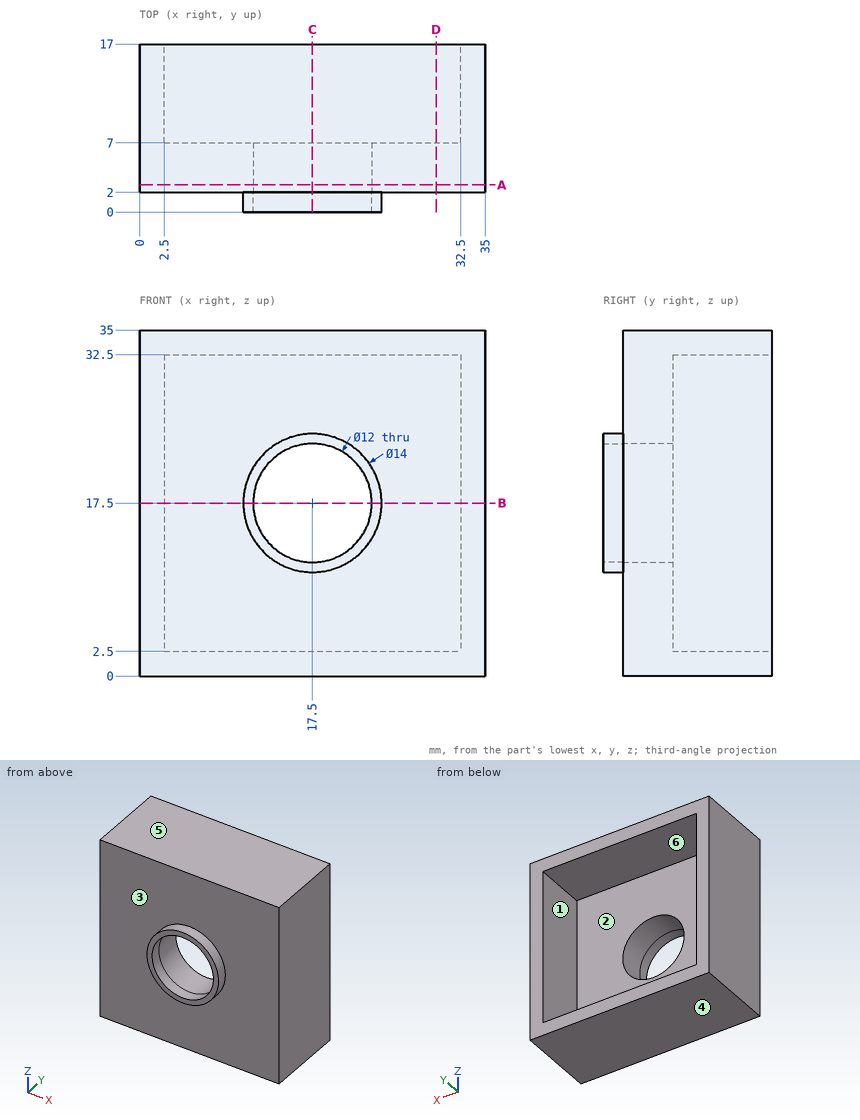
Print and shaded views of the part. All mm, measured from the part's lowest x, y and z. A direction names the side the tool comes from. Coordinates: 2 decimals unless noted, no trailing zeros. Order: outer loops, then holes, each group sorted by start corner. A loop starts at its lowest first (then second) coordinate and runs counter-clockwise, first axis right, second up. Notation, with made-up numbers: (-9.75, 31) -> (46.25, 31) arc R30 cw to (46.25, 54) -> close; hole circle Ø10 at (10, 88.25). An arc over 180 degrees is marked (long way). Answer as a JSON object with one key per item and string values. Group by question number.
1) Drill centre lines: L1, parallel to X at y = 12.25, z = 5.5; L2, parallel to X at y = 5.4, z = 17.5. Where is each one in solid material? Low to high.
2) Cut at D-D, the plane x = 30. Write the cut outline in (y, z), then the cut area to 3 significant figures.
3) Pull direction Z, two halves, no side cores. Call the marked faces 1, 2, 3 and 4: +Z half, -Z half, draft (parallel to the pull), parting line (faces both ways), or undercut.
4) Cut at A-A, the plane y = 2.75. Write the cut outline in (x, z), then the cut area to 3 significant figures.
5) Flat gauge pins, fed straight in: pin 1 (9 mm diameter, centred on x = 12.5, z = 12.5, fed in from +Y); pin 2 (1.5 mm diameter, centred on x = 27, z = 28, fed in from -Y). Where does each tip first touch, or does it go through?
6) Cut at C-C, the plane x = 17.5. Write the cut outline in (y, z), then the cut area to 3 significant figures.
7) Cut at B-B, the plane z = 17.5. Write the cut outline in (x, y).
8) Which spindle directions (+Z, -Z, +X, -X, +Y, -Y) get a long thin tool onto all of the face, cutting with end or side? Do the marked faces 5 and 6. Say none if no direction does.
Check values:
{
 "1": {"L1": "x = 0 to 2.5, 32.5 to 35", "L2": "x = 0 to 11.5, 23.5 to 35"},
 "2": {"outline": "(2, 0) -> (17, 0) -> (17, 2.5) -> (7, 2.5) -> (7, 32.5) -> (17, 32.5) -> (17, 35) -> (2, 35) -> close", "area": "225 mm²"},
 "3": {"face 1": "undercut", "face 2": "undercut", "face 3": "draft", "face 4": "-Z half"},
 "4": {"outline": "(0, 0) -> (35, 0) -> (35, 35) -> (0, 35) -> close; hole circle Ø12 at (17.5, 17.5)", "area": "1,110 mm²"},
 "5": {"pin 1": "stops at y = 7", "pin 2": "stops at y = 2"},
 "6": {"outline": "(0, 10.5) -> (2, 10.5) -> (2, 0) -> (17, 0) -> (17, 2.5) -> (7, 2.5) -> (7, 11.5) -> (0, 11.5) -> close; (0, 23.5) -> (7, 23.5) -> (7, 32.5) -> (17, 32.5) -> (17, 35) -> (2, 35) -> (2, 24.5) -> (0, 24.5) -> close", "area": "169 mm²"},
 "7": {"outline": "(0, 2) -> (10.5, 2) -> (10.5, 0) -> (11.5, 0) -> (11.5, 7) -> (2.5, 7) -> (2.5, 17) -> (0, 17) -> close; (23.5, 0) -> (24.5, 0) -> (24.5, 2) -> (35, 2) -> (35, 17) -> (32.5, 17) -> (32.5, 7) -> (23.5, 7) -> close"},
 "8": {"face 5": "+Z, +X, -X, +Y, -Y", "face 6": "+Y"}
}
